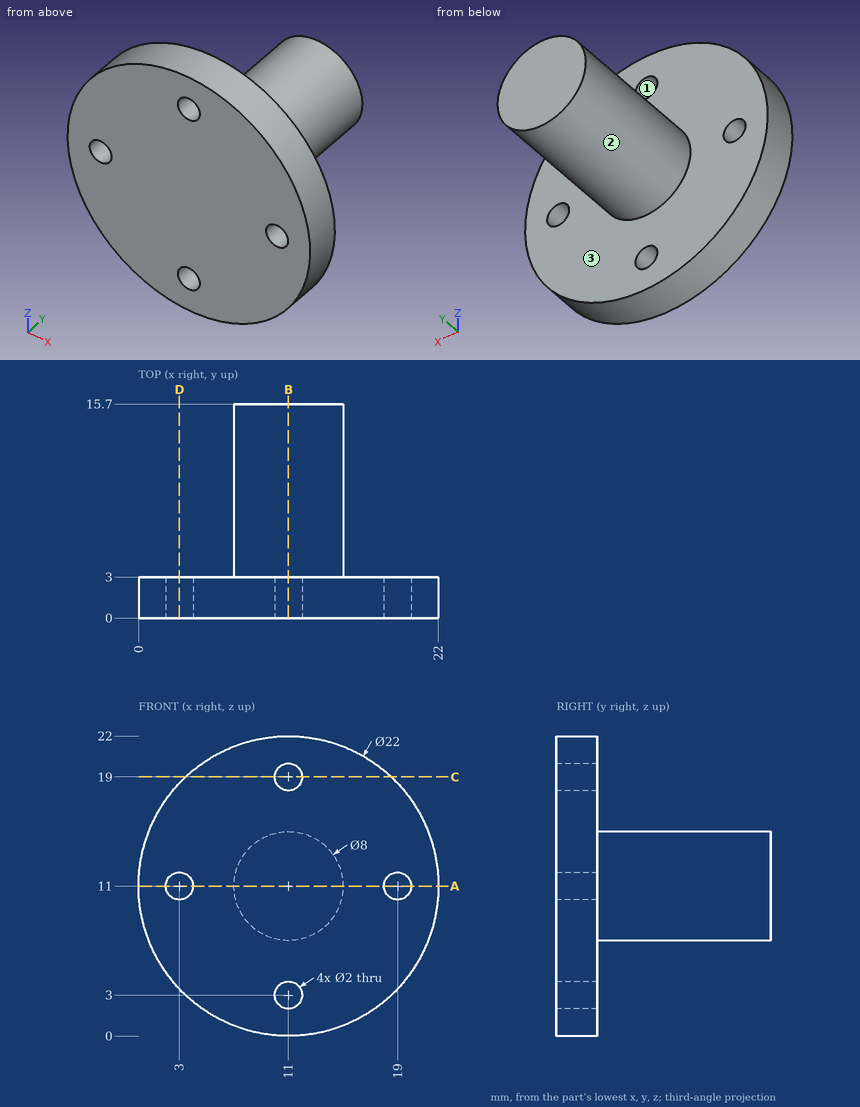
Drawing for the job (mm, zero at the part's lowest x, y, z). Give positions to 0.01 mm unless a question says otherwise; leave off trailing zeros. Order: outer loops, then holes, each group sorted by start corner. A loop starts at its lowest first (then second) coordinate and runs counter-clockwise, first axis right, second up. Notation, with made-up numbers: M 62,-5.5 L 104,-5.5 A22 cw 104,7.5 Z; hole C -5.75,56 d8. An arc over 180 degrees is marked long. Use a Markdown table: item, result. Add a question column.
(1) Saw through at A-A, the plane z = 11. Give the cut face in (x, y).
(2) Saw through at B-B, the plane x = 11. Give the cut face in (y, z).
(3) Saw through at D-D, the plane x = 3. Give the cut face in (y, z), and give its area (3 significant figures).
(4) Mould opens along Z. For the marked faces 1, 2 and 3 say: +Z half, -Z half, draft (parallel to the pull), parting line (faces both ways), or undercut.
(5) Saw through at C-C, the plane z = 19. Give the cut face in (x, y), and give its area (3 significant figures).
(6) Probe line 1 along X through (y, z) = (1.7, 11); line 2 along Y through (x, z) = (20.5, 6.25); line 3 along X through (y, z) = (10.5, 9.5). List the from-to ranges inside material, lowest first. Write a range as [from, to].
(7) Drop flat-ended pins along their axis: P1, Ø1.6, axis at x = 19, z = 11, coming from the +Y side; P2, Ø5, axis at x = 14.5, z = 5, coming from the +Y side; P3, Ø6, axis at y = 9.5, z = 16, coming from the +X side; P4, Ø1, axis at x = 13, y = 10, coming from the +Z side. Give the stop position or say it passes through.
Answer key:
| question | item | result |
|---|---|---|
| 1 | outline | M 0,0 L 2,0 L 2,3 L 0,3 Z; M 4,0 L 18,0 L 18,3 L 15,3 L 15,15.7 L 7,15.7 L 7,3 L 4,3 Z; M 20,0 L 22,0 L 22,3 L 20,3 Z |
| 2 | outline | M 0,0 L 3,0 L 3,2 L 0,2 Z; M 0,4 L 3,4 L 3,7 L 15.7,7 L 15.7,15 L 3,15 L 3,18 L 0,18 Z; M 0,20 L 3,20 L 3,22 L 0,22 Z |
| 3 | outline | M 0,3.45 L 3,3.45 L 3,10 L 0,10 Z; M 0,12 L 3,12 L 3,18.55 L 0,18.55 Z |
| 3 | area | 39.3 mm^2 |
| 4 | face 1 | undercut |
| 4 | face 2 | parting line |
| 4 | face 3 | draft |
| 5 | outline | M 3.45,0 L 10,0 L 10,3 L 3.45,3 Z; M 12,0 L 18.55,0 L 18.55,3 L 12,3 Z |
| 5 | area | 39.3 mm^2 |
| 6 | line 1 | [0, 2], [4, 18], [20, 22] |
| 6 | line 2 | [0, 3] |
| 6 | line 3 | [7.29, 14.71] |
| 7 | P1 | through |
| 7 | P2 | y = 3 |
| 7 | P3 | x = 14.46 |
| 7 | P4 | z = 14.71 |
